Autodesk Inventor part; units mm, degrees
ref_plane "Arbeitsebene1" through (5, -117, 0) normal (0, 1, 0) x (1, 0, 0)
ref_plane "YZ Plane" through (0, 0, 0) normal (1, 0, 0) x (0, 1, 0)
ref_plane "XZ Plane" through (0, 0, 0) normal (0, 1, 0) x (-1, 0, 0)
sketch "Skizze1" plane through (0, 0, 0) normal (0, 0, 1) x (1, 0, 0)
  line L0 (0, 0) -> (60, 0)
  line L1 (60, 0) -> (60, -150)
  line L2 (60, -150) -> (0, -150)
  line L3 (0, -150) -> (0, 0)
  circle A0 centre (30, -117) radius 9
  dimension "d0" = 60
  dimension "d1" = 150
  dimension "d2" = 18
extrude "Extrusion1" add sketch "Skizze1" along normal blind 10
sketch "Skizze2" plane through (0, -150, 0) normal (0, -1, 0) x (1, 0, 0)
  point P0 (0, 0)
  point P1 (6.5, 5)
  point P2 (53.5, 5)
hole "Bohrung1" at (6.5, -150, 5) at (53.5, -150, 5) direction (0, 1, 0) diameter 4.917 depth 50 tip angle 118
sketch "Skizze3" plane through (0, 0, 0) normal (0, 0, -1) x (-1, 0, 0)
  line L0 (-5, -117) -> (-55, -117)
  point P0 (0, 0)
ref_plane "Arbeitsebene1" through (5, -117, 0) normal (0, 1, 0) x (1, 0, 0)
split "Trennen1" plane through (5, -117, 0) removes the side toward (0, -1, 0)
properties part number "Steher oben Rohr"
Geometry check sheet. Reference: the model listing, model coordinates, mm. A direction names the side the tool comes from. Give positions to 0.01 mm unless a question says otherwise; leave off trailing zeros. Order: outer loops, then holes, each group sorted by start corner. A loop starts at its lowest first (then second) coordinate and runs counter-clockwise, first axis right, second up. Notation, with made-up numbers: (61.25, 8.25) - (97.25, 8.25) arc R21 cw to (97.25, 45.25) - close; hole circle Ø5 at (40, 36). An arc over 180 degrees is marked (long way). Write item = value, one per line. Start each with the question number.
1) Access from +Z, -Z, +X, -X, +Y, -Y to the whole of each face (thin tool, end or side, straight path). Record for faces 5 (the cylindrical face through (55.9, -108.38, 5.53)), 6 (the flat face through (60, -58, 5)).
2) Section check A-A (x = 30). Enter the section's corners in (y, z).
3) Gauge pin test, flat ends, axial feed: pin 1 Ø4.5 at (x, z) = (6.5, 5) entering from -Y; pin 2 Ø2 at (x, z) = (30.5, 2) entering from -Y. Record the tip position at first contact, or that the pin passes through.
4) Draft check along Z on faces 1 (the cylindrical face through (4.062, -108.381, 5.32)), 2 (the conical face through (6.52, -98.78, 5.43)), 3 (the flat face through (30, -58, 10)), 4 (the flat face through (49, -117, 5)). Enter one of: released by +Z, released by -Z, zero draft, split by the parting line, or undercut.
5) Scan lines: L1, parallel to X at y = -107.75, z = 5; L2, parallel to Z at x = 53.5, y = -109.25; L3, parallel to X at y = -109, z = 6. Record each from-to range of solid material in increasing order.
Geometry check:
q1.face_5 = -Y
q1.face_6 = +Z, -Z, +X, +Y, -Y
q2.outline = (-108, 0) - (0, 0) - (0, 10) - (-108, 10) - close
q3.pin_1 = -99.87
q3.pin_2 = -108.13
q4.face_1 = undercut
q4.face_2 = undercut
q4.face_3 = released by +Z
q4.face_4 = zero draft
q5.L1 = 0 to 4.04, 8.96 to 51.04, 55.96 to 60
q5.L2 = 0 to 2.54, 7.46 to 10
q5.L3 = 0 to 4.25, 8.75 to 25.88, 34.12 to 51.25, 55.75 to 60
